Geometry check sheet. Reference: the model listing, model coordinates, mm. Face numbers are marked on the shaded views. A direction names the side the tool comes from. Round coordinates to 2 decimals unless told otherwise and drop trailing zeros. Write each loop counter-clockwise with the first axis right and the second up, starting at its lowest first coordinate (ties: lowest second). Pieces come first, ordered by that corner, then holes. Notation, with made-up numbers: (19.25, 2) -> (53.25, 2) arc R31 ccw to (53.25, 34) -> close; hole circle Ø8 at (54, -8). An arc over 180 degrees is marked (long way). Return JSON: item names as keys, results as strings. Group by question number.
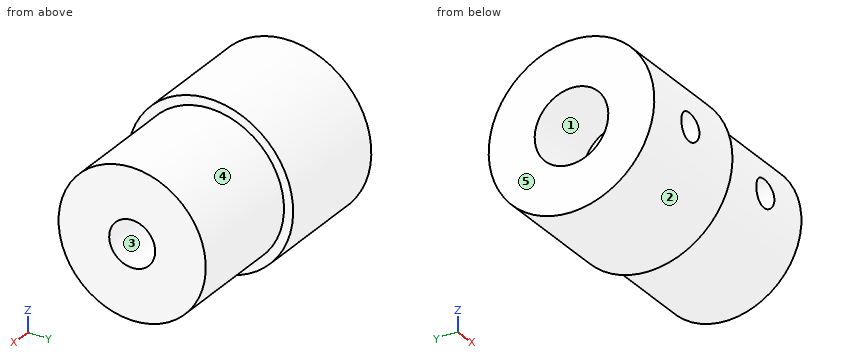
from build123d import *

# Parameters (mm, degrees)
ESQUISSE2_R             = 2.5
ENL_V_MAT_EXTRU_1_DEPTH = 29.948229652
ESQUISSE3_R             = 4
ENL_V_MAT_EXTRU_2_DEPTH = 8
ESQUISSE4_R             = 1.5
ENL_V_MAT_EXTRU_3_DEPTH = 29.948229652


with BuildPart() as part:
    # Esquisse1 → Révolution1 (revolve)
    with BuildSketch(Plane.XY, mode=Mode.PRIVATE) as r_volution1_sk:
        Polygon((0, 0), (0, 8), (-13, 8), (-13, 9), (-26, 9), (-26, 0), align=None)
    revolve(r_volution1_sk.sketch.rotate(Axis((0, 0, 0), (-1, 0, 0)), 90), axis=Axis((0, 0, 0), (-1, 0, 0)))

    # Esquisse2 → Enlèv. mat.-Extru.1 (cut, through all)
    with BuildSketch(Plane(origin=(0, 0, 0), x_dir=(0, 0, -1), z_dir=(1, 0, 0))):
        Circle(ESQUISSE2_R)
    extrude(amount=-ENL_V_MAT_EXTRU_1_DEPTH, mode=Mode.SUBTRACT)

    # Esquisse3 → Enlèv. mat.-Extru.2 (cut)
    with BuildSketch(Plane.ZY.offset(26)):
        Circle(ESQUISSE3_R)
    extrude(amount=-ENL_V_MAT_EXTRU_2_DEPTH, mode=Mode.SUBTRACT)

    # Esquisse4 → Enlèv. mat.-Extru.3 (cut, through all)
    with BuildSketch(Plane(origin=(0, 0, 0), x_dir=(1, 0, 0), z_dir=(0, 1, 0))):
        with Locations(Location((-20, 0, 0), (0, 0, 270))):
            Circle(ESQUISSE4_R)
        with Locations(Location((-6, 0, 0), (0, 0, 270))):
            Circle(ESQUISSE4_R)
    extrude(amount=-ENL_V_MAT_EXTRU_3_DEPTH, mode=Mode.SUBTRACT)


solid = part.part
1) Sectioned sample at C-C on z = -2. Enter the section's corners in (x, y), and give its area (3 significant figures).
2) Sectioned sample at A-A on z = 0. Enter the section's corners in (x, y), and give its area (4 significant figures).
3) Tool access check on the marked faces 1 and 2. Record the directions out of +Z, -Z, +X, -X, +Y, -Y that give a thin tool (end or side, any length) a straight path to the whole face; none if there is none.
4) Go/stop test with flat-tipped pins: P1, Ø4, axis at y = 0, z = 0, coming from the +X side; P2, Ø2.5, axis at y = 1.5, z = -1.5, coming from the -X side; P3, Ø1.5, axis at y = 2, z = 2, coming from the +X side; P4, Ø2, axis at x = -17.5, z = 2, coming from the +Y side. Record where each tip stops, or that it passes through.
5) Mould release check, pull along Y, two halves, no side actions. Record for the marked faces 3, 4 and 5: +Y half, -Y half, draft (parallel to the pull), parting line (faces both ways), or undercut.
6) Sectioned sample at B-B on y = 0. Enter the section's corners in (x, z).
7) Material ranges on probe 1 along X at (y, z) = (-6.25, 0); probe 2 along Z at (x, y) = (-20, -5.25); probe 3 along Z at (x, y) = (-22.5, -2.5), recorded low to high. Write a range as [from, to].
8) Sectioned sample at D-D on x = -15.25. Enter the section's corners in (y, z), and give its area (3 significant figures).
Evaluation:
{
 "1": {"outline": "(-26, -8.77) -> (-13, -8.77) -> (-13, -7.75) -> (0, -7.75) -> (0, -1.5) -> (-18, -1.5) -> (-18, -3.46) -> (-26, -3.46) -> close; (-26, 3.46) -> (-18, 3.46) -> (-18, 1.5) -> (0, 1.5) -> (0, 7.75) -> (-13, 7.75) -> (-13, 8.77) -> (-26, 8.77) -> close", "area": "320 mm2"},
 "2": {"outline": "(-26, -9) -> (-21.5, -9) -> (-21.5, -4) -> (-26, -4) -> close; (-26, 4) -> (-18, 4) -> (-18, 2.5) -> (0, 2.5) -> (0, 8) -> (-13, 8) -> (-13, 9) -> (-26, 9) -> close; (-18.5, -9) -> (-13, -9) -> (-13, -8) -> (-7.5, -8) -> (-7.5, -2.5) -> (-18, -2.5) -> (-18, -4) -> (-18.5, -4) -> close; (-4.5, -8) -> (0, -8) -> (0, -2.5) -> (-4.5, -2.5) -> close", "area": "256.5 mm2"},
 "3": {"face 1": "-X", "face 2": "+X, -X"},
 "4": {"P1": "passes through", "P2": "stops at x = -18", "P3": "stops at x = 0", "P4": "stops at y = 8.94"},
 "5": {"face 3": "undercut", "face 4": "parting line", "face 5": "draft"},
 "6": {"outline": "(-26, -9) -> (-13, -9) -> (-13, -8) -> (0, -8) -> (0, -2.5) -> (-18, -2.5) -> (-18, -4) -> (-26, -4) -> close; (-26, 4) -> (-18, 4) -> (-18, 2.5) -> (0, 2.5) -> (0, 8) -> (-13, 8) -> (-13, 9) -> (-26, 9) -> close"},
 "7": {"probe 1": "x = [-26, -21.5], [-18.5, -7.5], [-4.5, 0]", "probe 2": "z = [-7.31, -1.5], [1.5, 7.31]", "probe 3": "z = [-8.65, -3.12], [3.12, 8.65]"},
 "8": {"outline": "circle Ø18 at (0, 0); hole circle Ø5 at (0, 0)", "area": "235 mm2"}
}
